Can you work these out from the model? Positions are in its coordinate system, mm. A direction names the side the tool comes from. Coordinates: 2 decimals unless noted, no trailing zeros. Order: outer loops, then holes, each group sorted by start corner. A loop starts at its lowest first (then second) coordinate and runs counter-clockwise, first axis right, second up. Notation, with made-up numbers: (-14.75, -9) -> (2.25, -9) arc R23 ccw to (2.25, 0) -> close; hole circle Ø7 at (75.25, -24). An arc over 180 degrees is marked (long way). Return JSON: item names as keys, results as strings. Group by question number.
1) If I drill on probe 1 along Z at (x, y) = (619.5, 17.5); probe 2 along Y at (x, z) = (454.5, -20); probe 3 along X at (y, z) = (-28, -27.5), over which ranges is the centre line in solid material (lowest first)? Write a range as from..to.
2) For pin 1 (13.5 mm diameter, centred on x = 481, z = -7, fed in from +Y); pin 2 (22 mm diameter, centred on x = 477, y = 2, fed in from -Z), each with a flat end and sliding along its axis, tell me the tip position at first contact or that it passes through.
3) For faces 1 (the flat face through (16, -15, 13)), 2 (the flat face through (545, -3, 11.943)), which set-ups out of +Z, -Z, +X, -X, +Y, -Y let a thin tool reach every point of the face, with its end or its side?
4) If we section it at C-C, the plane y = -8.5: Please give me the cut outline in (x, z), then the cut area to 3 significant figures.
5) If we section it at A-A, the plane x = 945: Please give me the cut outline in (y, z), then the cut area to 3 significant figures.
from build123d import *

# Parameters (mm, degrees)
F1_DEPTH = 1104.9
F2_SIZE2 = 50.79999
F2_SIZE  = 50.79999


# Not quite as in the source:
# - a fillet or chamfer is up to 0.001 mm smaller than in the source, because OpenCascade refuses the exact size


with BuildPart() as f1:
    # F0 (on Right) → F1 (new body)
    with BuildSketch(Plane.YZ):
        Polygon((-30.9975855052, -32.5072072446), (-24.6475855052, -32.5072072446), (-24.6475855052, 11.9427927554), (19.8024144948, 11.9427927554), (19.8024144948, 18.2927927554), (-30.9975855052, 18.2927927554), align=None)
    extrude(amount=F1_DEPTH)

    # F2 (size 50.8 and 50.8 in the source; OpenCascade refuses exactly that, so slightly less here)
    f2_edges = [f1.edges().sort_by_distance(p)[0] for p in [
        (1104.9, 19.802414, 15.117793),
        (0, 19.802414, 15.117793),
    ]]
    chamfer(f2_edges, length=F2_SIZE, length2=F2_SIZE2)


solid = f1.part
Result sheet:
{
 "1": {"probe 1": "z = 11.94..18.29", "probe 2": "y = -31..-24.65", "probe 3": "x = 3..1101.9"},
 "2": {"pin 1": "stops at y = -24.65", "pin 2": "stops at z = 11.94"},
 "3": {"face 1": "+Z, -Z, -X, +Y", "face 2": "-Z, +X, -X, +Y"},
 "4": {"outline": "(22.5, 11.94) -> (1082.4, 11.94) -> (1082.4, 18.29) -> (22.5, 18.29) -> close", "area": "6,730 mm2"},
 "5": {"outline": "(-31, -32.51) -> (-24.65, -32.51) -> (-24.65, 11.94) -> (19.8, 11.94) -> (19.8, 18.29) -> (-31, 18.29) -> close", "area": "605 mm2"}
}
